Print and shaded views of the part. All mm, measured from the part's lowest x, y and z. A direction names the side the tool comes from. Give positions to 0.01 mm unless a question says otherwise; leave off trailing zeros. Loops run counter-clockwise (first coordinate to the right, second up) from the corner with the lowest first, then second, coordinate; pieces in that order, holes last.
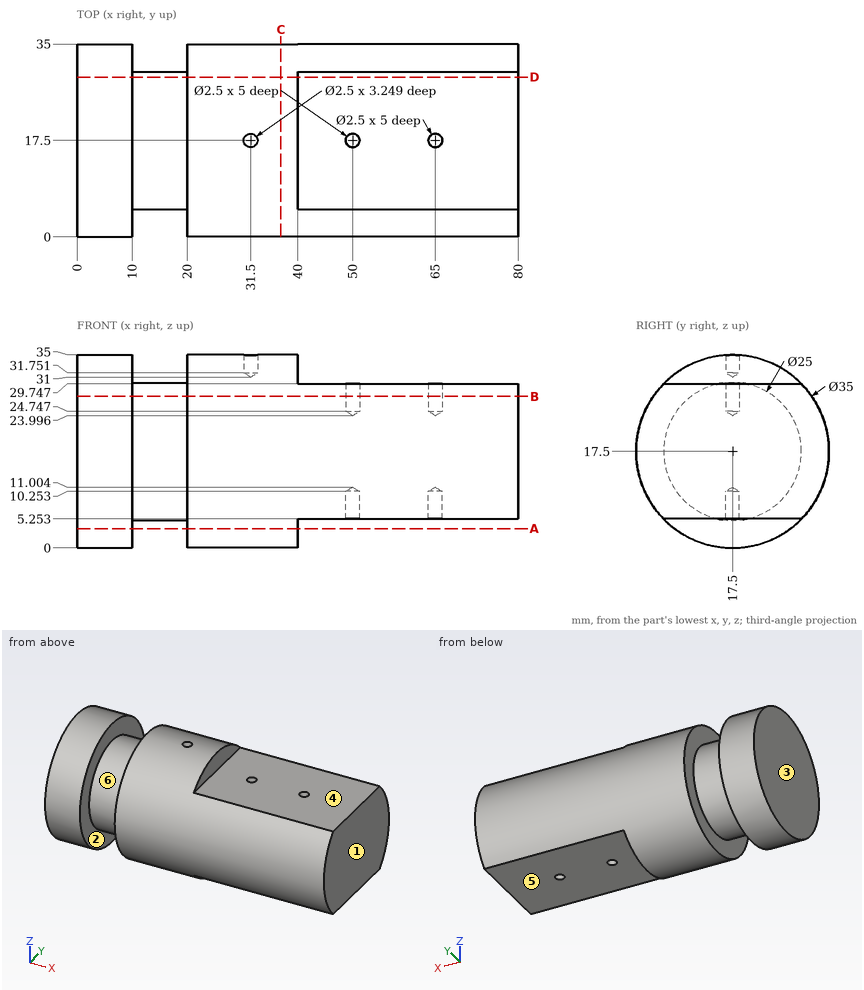
1. Saw through at C-C, the plane x = 37. List the corners of the cut face in (y, z), and give its area (3 significant figures).
Responses:
outline: circle Ø35 at (17.5, 17.5)
area: 962 mm2
2. Pull direction X, two halves, no side cores. Call the marked faces 1, 2 and 3: released by +X, released by -X, zero draft, split by the parting line, or undercut.
Responses:
face 1: released by +X
face 2: undercut
face 3: released by -X
3. Tool access for the marked faces 4, 5 and 6: list every direction of +Z, -Z, +X, -X, +Y, -Y with a clear straight run to the whole face (end or side of a thin tool).
Responses:
face 4: +Z, +X, +Y, -Y
face 5: -Z, +X, +Y, -Y
face 6: none
4. Probe line 1 along X through (y, z) = (3.5, 24.5); line 2 along X through (y, z) = (27, 31.5); line 3 along Z through (x, y) = (70.5, 29.5). List the from-to ranges inside material, lowest first.
Responses:
line 1: x = 0 to 10, 20 to 80
line 2: x = 0 to 10, 20 to 40
line 3: z = 5.25 to 29.75
5. Saw through at D-D, the plane y = 29. List the corners of the cut face in (x, z), and give its area (3 significant figures).
Responses:
outline: (0, 4.31) - (10, 4.31) - (10, 12.6) - (20, 12.6) - (20, 4.31) - (40, 4.31) - (40, 5.25) - (80, 5.25) - (80, 29.75) - (40, 29.75) - (40, 30.69) - (20, 30.69) - (20, 22.4) - (10, 22.4) - (10, 30.69) - (0, 30.69) - close
area: 1,870 mm2
6. Saw through at B-B, the plane z = 27.5. List the corners of the cut face in (x, y), and give its area (3 significant figures).
Responses:
outline: (0, 3.14) - (10, 3.14) - (10, 10) - (20, 10) - (20, 3.14) - (80, 3.14) - (80, 31.86) - (20, 31.86) - (20, 25) - (10, 25) - (10, 31.86) - (0, 31.86) - close; hole circle Ø2.5 at (50, 17.5); hole circle Ø2.5 at (65, 17.5)
area: 2,150 mm2
7. Saw through at A-A, the plane z = 3.5. List the corners of the cut face in (x, y).
Responses:
outline: (0, 7) - (10, 7) - (10, 28) - (0, 28) - close; (20, 7) - (40, 7) - (40, 28) - (20, 28) - close
8. Drop flat-ended pins along their axis: pin 1 (1 mm diameter, centred on y = 14.5, z = 30.5, fed in from +X); pin 2 (7.5 mm diameter, centred on x = 64.5, y = 17, fed in from +Z); pin 3 (2 mm diameter, centred on x = 36.5, y = 8.5, fed in from -Z) (1 decimal). Give the stop position or say it passes through.
Responses:
pin 1: stops at x = 40
pin 2: stops at z = 29.75
pin 3: stops at z = 1.9
